Here's the drawing with two shaded views (mm, measured from the low corner). I have some questions. Round coordinates to 2 decimals unless told otherwise and drop trailing zeros. Loops run counter-clockwise (first coordinate to the right, second up) from the corner with the lowest first, then second, coordinate; pieces in that order, holes last.
(1) I want a section at B-B on z = 3.75. Write out the boundary of the cut face in (x, y) (3 decimals), plus the area to 3 significant figures.
(2) Will these pins go through, and if not, where does the flat tip stop? pin 1 Ø4 at (x, z) = (7, 4.5) entering from -Y; pin 2 Ø1 at (x, z) = (5, 6) entering from +Y; pin 3 Ø2 at (y, z) = (73.5, 3.5) entering from +X; pin 4 Ø1.5 at (x, y) = (8.5, 34.5) entering from -Z.
(3) If I drill on line 1 along Y through (x, z) = (4.25, 5); line 2 along X through (y, z) = (41, 5); line 3 along X through (y, z) = (57, 0.5), over which ranges is the centre line in solid material (lowest first)?
(4) I want a section at D-D on z = 8.75. Write out the boundary of the cut face in (x, y).
(5) Thinking about a two-plate mould opening in X: for the marked faces 1, 2 and 3, which applies, released by +X, released by -X, zero draft, split by the parting line, or undercut?
(6) I want a section at A-A on x = 5.25. Write out the boundary of the cut face in (y, z) (3 decimals), plus the area to 3 significant figures.
(7) I want a section at C-C on y = 47. Write out the boundary of the cut face in (x, z) (3 decimals), plus the area to 3 significant figures.
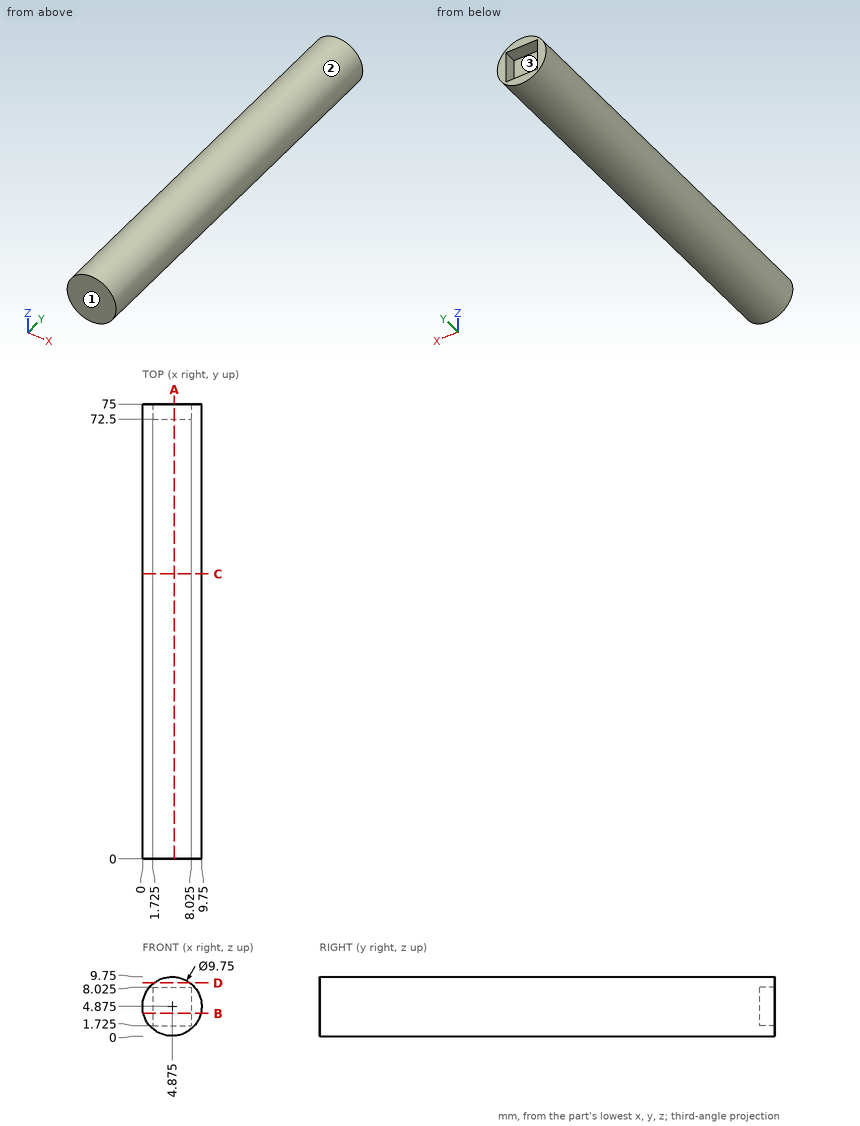
Filled sheet:
1. outline: (0.132, 0) - (9.618, 0) - (9.618, 75) - (8.025, 75) - (8.025, 72.5) - (1.725, 72.5) - (1.725, 75) - (0.132, 75) - close
1. area: 696 mm2
2. pin 1: stops at y = 0
2. pin 2: stops at y = 72.5
2. pin 3: stops at x = 9.74
2. pin 4: stops at z = 0.94
3. line 1: y = 0 to 72.5
3. line 2: x = 0 to 9.75
3. line 3: x = 2.72 to 7.03
4. outline: (1.92, 0) - (7.83, 0) - (7.83, 75) - (1.92, 75) - close
5. face 1: zero draft
5. face 2: split by the parting line
5. face 3: undercut
6. outline: (0, 0.014) - (75, 0.014) - (75, 1.725) - (72.5, 1.725) - (72.5, 8.025) - (75, 8.025) - (75, 9.736) - (0, 9.736) - close
6. area: 713 mm2
7. outline: circle Ø9.75 at (4.875, 4.875)
7. area: 74.7 mm2
